The model under review builds one solid part; all positions refer to its coordinate system, in mm. Face numbers are marked on the shaded views. Round coordinates to 2 decimals unless told otherwise and drop trailing zeros. Order: outer loops, then holes, each group sorted by start corner. A loop starts at its lowest first (then second) coordinate and runs counter-clockwise, first axis right, second up. Notation, with made-up numbers: M -1,20.5 L 50,20.5 A27 cw 50,36.5 Z; hole C -35,45.25 d6. An arc over 180 degrees is marked long. Answer as a JSON object with one key per item and string values. Group by question number.
1. To check wall thickness, follow probe 1 along X at (y, z) = (80, 4); probe 2 along X at (y, z) = (82, 0.45); probe 3 along Y at (x, z) = (3, 1.3). State the ranges of each line that lie inside material, in increasing order. Write a range as [from, to].
2. Mouldability with a two-part tool opening along X and no side actions: class the marked faces 1, 2 and 3 as released by +X, released by -X, zero draft, split by the parting line, or undercut.
3. Add section B-B on y = 94.5. State the section outline as (x, z) points, and give its area (3 significant figures).
4. Clearance check with flat-ended pins moving along their axes: P1, Ø5, axis at x = 10, y = 91.5, coming from the -Z side; P2, Ø3, axis at x = 37, z = 3.5, coming from the +Y side; P3, Ø1, axis at y = 82.5, z = 3, coming from the -X side. State where each tip first meets the part, or that it passes through.
5. Add section A-A on z = 1.5. State the section outline as (x, y) points (3 decimals), and give its area (3 significant figures).
6. Add section C-C on x = 29.5. State the section outline as (y, z) points, and give its area (3 significant figures).
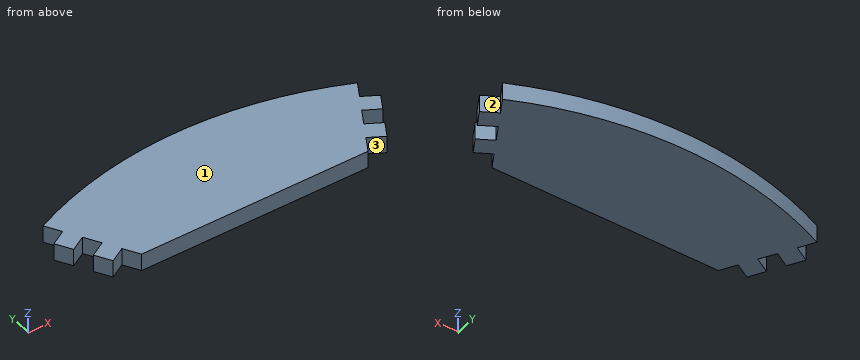
```python
from build123d import *

# Parameters (mm, degrees)
BOSS_EXTRUDE1_DEPTH = 5


with BuildPart() as part:
    # Sketch1 → Boss-Extrude1 (new body)
    with BuildSketch(Plane.XY):
        with BuildLine():
            Line((-32.85, 77.986683936), (32.85, 77.986683936))
            Line((32.85, 77.986683936), (35.403, 82.408609648))
            Line((35.403, 82.408609648), (39.733127019, 79.908609648))
            Line((39.733127019, 79.908609648), (42.286127019, 84.330535359))
            Line((42.286127019, 84.330535359), (37.956, 86.830535359))
            Line((37.956, 86.830535359), (40.509, 91.252461071))
            Line((40.509, 91.252461071), (44.839127019, 88.752461071))
            Line((44.839127019, 88.752461071), (47.392127019, 93.174386783))
            Line((47.392127019, 93.174386783), (43.062, 95.674386783))
            Line((43.062, 95.674386783), (45.615, 100.096312495))
            ThreePointArc((45.615, 100.096312495), (0, 110), (-45.615, 100.096312495))
            Line((-45.615, 100.096312495), (-43.062, 95.674386783))
            Line((-43.062, 95.674386783), (-47.392127019, 93.174386783))
            Line((-47.392127019, 93.174386783), (-44.839127019, 88.752461071))
            Line((-44.839127019, 88.752461071), (-40.509, 91.252461071))
            Line((-40.509, 91.252461071), (-37.956, 86.830535359))
            Line((-37.956, 86.830535359), (-42.286127019, 84.330535359))
            Line((-42.286127019, 84.330535359), (-39.733127019, 79.908609648))
            Line((-39.733127019, 79.908609648), (-35.403, 82.408609648))
            Line((-35.403, 82.408609648), (-32.85, 77.986683936))
        make_face()
    extrude(amount=BOSS_EXTRUDE1_DEPTH)


solid = part.part
```
Recorded:
{
 "1": {"probe 1": "x = [-39.79, -39.57], [-34.01, 34.01], [39.57, 39.79]", "probe 2": "x = [-40.94, -36.11], [-35.17, 35.17], [36.11, 40.94]", "probe 3": "y = [77.99, 109.96]"},
 "2": {"face 1": "zero draft", "face 2": "released by +X", "face 3": "undercut"},
 "3": {"outline": "M -45.1,0 L 45.1,0 L 45.1,5 L -45.1,5 Z", "area": "451 mm²"},
 "4": {"P1": "stops at z = 0", "P2": "stops at y = 104.11", "P3": "stops at x = -41.52"},
 "5": {"outline": "M -47.392,93.174 L -44.839,88.752 L -40.509,91.252 L -37.956,86.831 L -42.286,84.331 L -39.733,79.909 L -35.403,82.409 L -32.85,77.987 L 32.85,77.987 L 35.403,82.409 L 39.733,79.909 L 42.286,84.331 L 37.956,86.831 L 40.509,91.252 L 44.839,88.752 L 47.392,93.174 L 43.062,95.674 L 45.615,100.096 A110 ccw -45.615,100.096 L -43.062,95.674 Z", "area": "2,440 mm²"},
 "6": {"outline": "M 77.99,0 L 105.97,0 L 105.97,5 L 77.99,5 Z", "area": "140 mm²"}
}
